Part model, mm, in its own coordinate system. Face numbers are marked on the shaded views. Give positions to 0.01 mm unless a question says otherwise; leave off trailing zeros. Loops run counter-clockwise (first coordinate to the right, second up) from the corner with the lowest first, then second, coordinate; pieces in that order, holes last. Notation, with made-up numbers: M 41.25,2.25 L 77.25,2.25 A21 cw 77.25,19.25 Z; hole C 80.5,67.25 d10. An arc over 180 degrees is marked long. Answer in a Markdown table with one row per item.
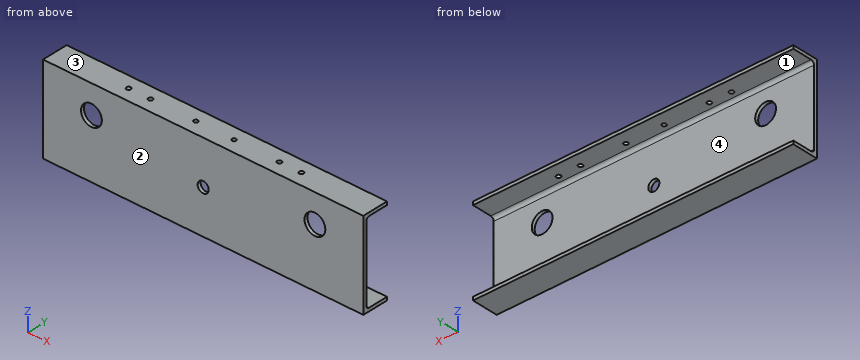
from build123d import *

# Parameters (mm, degrees)
F1_DEPTH = 923.925
F3_D     = 12.7
F3_DEPTH = 30
F5_D     = 60
F5_DEPTH = 30
F6_D     = 32
F6_DEPTH = 30
F7_D     = 12
F7_DEPTH = 30


with BuildPart() as f1:
    # F0 (on Right) → F1 (new body)
    with BuildSketch(Plane.YZ):
        with BuildLine():
            Line((-26.569311, 131.535714), (-26.569311, -122.464286))
            Line((-26.569311, -122.464286), (49.630689, -122.464286))
            Line((49.630689, -122.464286), (49.630689, -112.939286))
            Line((49.630689, -112.939286), (-7.519311, -112.939286))
            ThreePointArc((-7.519311, -112.939286), (-14.254503, -110.149478), (-17.044311, -103.414286))
            Line((-17.044311, -103.414286), (-17.044311, 112.485714))
            ThreePointArc((-17.044311, 112.485714), (-14.254503, 119.220906), (-7.519311, 122.010714))
            Line((-7.519311, 122.010714), (49.630689, 122.010714))
            Line((49.630689, 122.010714), (49.630689, 131.535714))
            Line((49.630689, 131.535714), (-26.569311, 131.535714))
        make_face()
    extrude(amount=F1_DEPTH)

    # F3
    with Locations(Plane.XY.offset(131.535714)):
        with Locations((212.725, 11.530689), (276.225, 11.530689), (647.7, 11.530689), (711.2, 11.530689)):
            Hole(F3_D / 2, depth=F3_DEPTH)

    # F5
    with Locations(Plane.XZ.offset(26.569311)):
        with Locations((139.7, 48.985714), (784.225, 48.985714)):
            Hole(F5_D / 2, depth=F5_DEPTH)

    # F6
    with Locations(Plane.XZ.offset(26.569311)):
        with Locations((461.9625, 4.535714)):
            Hole(F6_D / 2, depth=F6_DEPTH)

    # F7
    with Locations(Plane.XY.offset(131.535714)):
        with Locations((406.9625, 11.530689), (516.9625, 11.530689)):
            Hole(F7_D / 2, depth=F7_DEPTH)


solid = f1.part
(1) Saw through at B-B (x = 139.7). Write the cut outline in (y, z) (3 decimals), plus the area to 3 significant figures.
Recorded:
| item | result |
|---|---|
| outline | M -26.569,-122.464 L 49.631,-122.464 L 49.631,-112.939 L -7.519,-112.939 A9.525 cw -17.044,-103.414 L -17.044,18.986 L -26.569,18.986 Z; M -26.569,78.986 L -17.044,78.986 L -17.044,112.486 A9.525 cw -7.519,122.011 L 49.631,122.011 L 49.631,131.536 L -26.569,131.536 Z |
| area | 3,160 mm^2 |
(2) Pin check, flat tips, straight feed: pin 1 Ø10 at (x, y) = (711.2, 11.53) entering from +Z; pin 2 Ø3 at (x, z) = (237, 18) entering from +Y. Stop position of each tip, or through.
Recorded:
| item | result |
|---|---|
| pin 1 | stops at z = -112.94 |
| pin 2 | stops at y = -17.04 |
(3) Pull direction Z, two halves, no side cores. Call the marked faces 1, 2, 3 and 4: +Z half, -Z half, draft (parallel to the pull), parting line (faces both ways), or undercut.
Recorded:
| item | result |
|---|---|
| face 1 | undercut |
| face 2 | draft |
| face 3 | +Z half |
| face 4 | undercut |
(4) Saw through at C-C (z = 40.5). Write the cut outline in (x, y) (3 decimals), plus the area to 3 significant figures.
Recorded:
| item | result |
|---|---|
| outline | M 0,-26.569 L 110.925,-26.569 L 110.925,-17.044 L 0,-17.044 Z; M 168.475,-26.569 L 755.45,-26.569 L 755.45,-17.044 L 168.475,-17.044 Z; M 813,-26.569 L 923.925,-26.569 L 923.925,-17.044 L 813,-17.044 Z |
| area | 7,700 mm^2 |
(5) Saw through at D-D (x = 631). Write the cut outline in (y, z) (3 decimals), plus the area to 3 significant figures.
Recorded:
| item | result |
|---|---|
| outline | M -26.569,-122.464 L 49.631,-122.464 L 49.631,-112.939 L -7.519,-112.939 A9.525 cw -17.044,-103.414 L -17.044,112.486 A9.525 cw -7.519,122.011 L 49.631,122.011 L 49.631,131.536 L -26.569,131.536 Z |
| area | 3,730 mm^2 |
(6) Saw through at A-A (y = 40.5). Write the cut outline in (x, z) (3 decimals), plus the area to 3 significant figures.
Recorded:
| item | result |
|---|---|
| outline | M 0,-122.464 L 923.925,-122.464 L 923.925,-112.939 L 0,-112.939 Z; M 0,122.011 L 923.925,122.011 L 923.925,131.536 L 0,131.536 Z |
| area | 17,600 mm^2 |
(7) Drill centre lines: line 1 along Z through (x, y) = (244, -7); line 2 along Z through (x, y) = (138.5, -23); line 3 along Y through (x, z) = (271.5, 30.5). Where is each one in solid material? Low to high.
Recorded:
| item | result |
|---|---|
| line 1 | z = -122.46 to -112.94, 122.01 to 131.54 |
| line 2 | z = -122.46 to 19.01, 78.96 to 131.54 |
| line 3 | y = -26.57 to -17.04 |
